Geometry: see drawing. Coordinates: mm, zero at the bounding-box minimum. Give positions to 0.01 mm unless a question says otherwise; leave off trailing zeros. Order: outer loops, then holes, each group sorted by start corner. A loop starts at its lowest first (then second) coordinate and runs counter-clockwise, first axis right, second up. Notation, with made-up numbers: M -3,81 L 51,81 A15 ccw 51,85 Z; hole C 20,-32 d5. An arc over 180 degrees is marked long. Use a Markdown table: item, result.
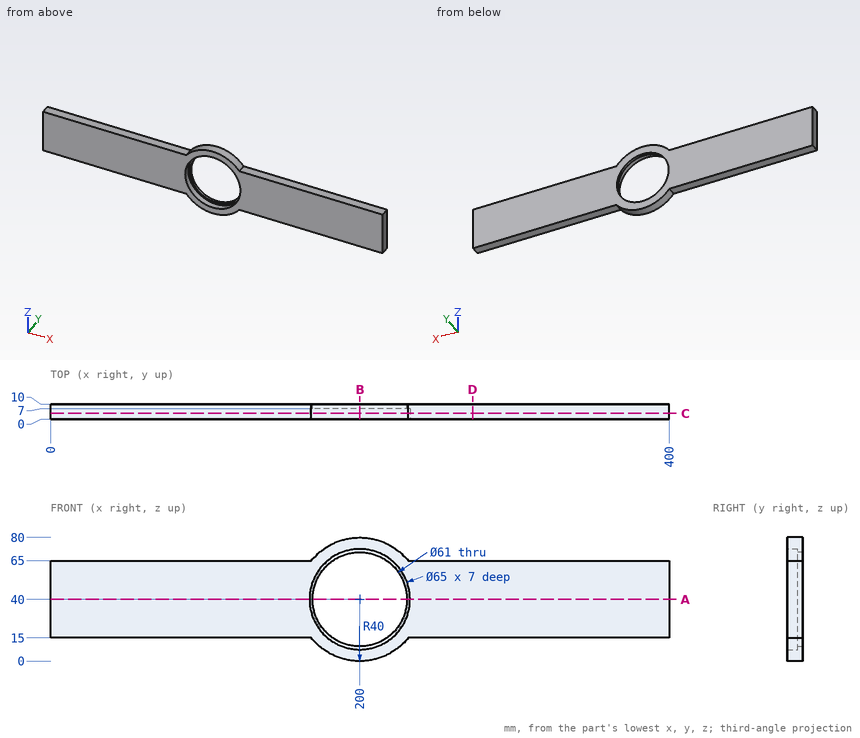
1) Cut plane B-B on x = 200. Return loops of the section in (y, z).
Response values:
| item | result |
|---|---|
| outline | M 0,0 L 10,0 L 10,9.5 L 7,9.5 L 7,7.5 L 0,7.5 Z; M 0,72.5 L 7,72.5 L 7,70.5 L 10,70.5 L 10,80 L 0,80 Z |
2) Material intervals for line 1 (X direction, y = 4.5, z = 40); line 2 (X direction, y = 7.7, z = 40); line 3 (Z direction, x = 329.5, y = 1.25), sorted ascending. Write a range as from..to.
Response values:
| item | result |
|---|---|
| line 1 | x = 0..167.5, 232.5..400 |
| line 2 | x = 0..169.5, 230.5..400 |
| line 3 | z = 15..65 |
3) Cut plane D-D on x = 273. Return loops of the section in (y, z).
Response values:
| item | result |
|---|---|
| outline | M 0,15 L 10,15 L 10,65 L 0,65 Z |
4) First-contact query: pin 1 Ø5 at (x, z) = (69.5, 47) entering from -Y; pin 2 Ø5 at (x, y) = (45, 4) entering from -Z; pin 3 Ø3 at (x, y) = (79.5, 6.5) entering from +Z. Flat tips, straight axial feed; report the tip coordinate or a pass-through.
Response values:
| item | result |
|---|---|
| pin 1 | stops at y = 0 |
| pin 2 | stops at z = 15 |
| pin 3 | stops at z = 65 |
5) Cut plane A-A on z = 40. Return loops of the section in (x, y).
Response values:
| item | result |
|---|---|
| outline | M 0,0 L 167.5,0 L 167.5,7 L 169.5,7 L 169.5,10 L 0,10 Z; M 230.5,7 L 232.5,7 L 232.5,0 L 400,0 L 400,10 L 230.5,10 Z |
6) Cut plane C-C on y = 4. Return loops of the section in (x, z).
Response values:
| item | result |
|---|---|
| outline | M 0,15 L 168.78,15 A40 ccw 231.22,15 L 400,15 L 400,65 L 231.22,65 A40 ccw 168.78,65 L 0,65 Z; hole C 200,40 d65 |
